Geometry check sheet. Reference: the model listing, model coordinates, mm. Round coordinates to 2 decimals unless told otherwise and drop trailing zeros. Write each loop counter-clockwise with the first axis right and the second up, starting at its lowest first coordinate (ties: lowest second). Pieces come first, ordered by that corner, then holes. Notation, with made-up numbers: M 64.5,-36.75 L 80.5,-36.75 A17 ccw 80.5,-15.75 Z; hole C 54.5,-18 d5. An arc over 180 degrees is marked long. Put each result on its own line as item: value. Start each with the question number.
(1) Section check A-A on y = 1. Record the cut outline in (x, z).
(2) Gauge pin test, flat ends, axial feed: pin 1 (0.5 mm diameter, centred on y = -1, z = -1.5, fed in from -X); pin 2 (0.7 mm diameter, centred on x = 1.5, y = 6, fed in from -Z); pin 3 (0.7 mm diameter, centred on x = 1.5, y = -1, fed in from +Z). Record the tip position at first contact, or that the pin passes through.
(3) Section check D-D on y = -1.5. Record the cut outline in (x, z), then the cut area to 3 significant figures.
(4) Material ranges on probe 1 along X at (y, z) = (7, -1.35); probe 2 along Y at (x, z) = (1.45, -1.65); probe 3 along Z at (x, y) = (1.25, 7.5), recorded low to high.
(5) Section check B-B on x = 1.05. Record the cut outline in (y, z).
(6) Section check C-C on z = -1.4. Record the cut outline in (x, y), then the cut area to 3 significant figures.
from build123d import *

# Parameters (mm, degrees)
BOSS_EXTRUDE1_DEPTH = 2.54
SKETCH2_W           = 0.635
SKETCH2_H           = 0.635
BOSS_EXTRUDE2_DEPTH = 5.842
SKETCH5_W           = 0.635
SKETCH5_H           = 0.635
BOSS_EXTRUDE3_DEPTH = 3.048


with BuildPart() as part:
    # Sketch1 → Boss-Extrude1 (new body)
    with BuildSketch(Plane(origin=(0, 0, 0), x_dir=(1, 0, 0), z_dir=(0, 1, 0))):
        Polygon((0.381, 0), (0, 0.762), (0, 1.6764), (0.381, 2.4384), (2.159, 2.4384), (2.54, 1.6764), (2.54, 0.762), (2.159, 0), align=None)
    extrude(amount=BOSS_EXTRUDE1_DEPTH)

    # Sketch2 → Boss-Extrude2 (add)
    with BuildSketch(Plane(origin=(0, 2.54, 0), x_dir=(1, 0, 0), z_dir=(0, 1, 0))):
        with Locations((1.27, 1.2192)):
            Rectangle(SKETCH2_W, SKETCH2_H)
    extrude(amount=BOSS_EXTRUDE2_DEPTH)

    # Sketch5 → Boss-Extrude3 (add)
    with BuildSketch(Plane.XZ):
        with Locations((1.27, -1.2192)):
            Rectangle(SKETCH5_W, SKETCH5_H)
    extrude(amount=BOSS_EXTRUDE3_DEPTH)


solid = part.part
Answers follow:
1. outline: M 0,-1.68 L 0.38,-2.44 L 2.16,-2.44 L 2.54,-1.68 L 2.54,-0.76 L 2.16,0 L 0.38,0 L 0,-0.76 Z
2. pin 1: stops at x = 0.95
2. pin 2: stops at z = -1.54
2. pin 3: stops at z = -0.9
3. outline: M 0.95,-1.54 L 1.59,-1.54 L 1.59,-0.9 L 0.95,-0.9 Z
3. area: 0.403 mm^2
4. probe 1: x = 0.95 to 1.59
4. probe 2: y = 0 to 2.54
4. probe 3: z = -1.54 to -0.9
5. outline: M -3.05,-1.54 L 0,-1.54 L 0,-2.44 L 2.54,-2.44 L 2.54,-1.54 L 8.38,-1.54 L 8.38,-0.9 L 2.54,-0.9 L 2.54,0 L 0,0 L 0,-0.9 L -3.05,-0.9 Z
6. outline: M 0,0 L 0.95,0 L 0.95,-3.05 L 1.59,-3.05 L 1.59,0 L 2.54,0 L 2.54,2.54 L 1.59,2.54 L 1.59,8.38 L 0.95,8.38 L 0.95,2.54 L 0,2.54 Z
6. area: 12.1 mm^2
